Geometry check sheet. Reference: the model listing, model coordinates, mm. A direction names the side the tool comes from. Give positions to 0.01 mm unless a question says otherwise; leave off trailing zeros. Order: outer loops, then holes, each group sorted by start corner. A loop starts at its lowest first (then second) coordinate and runs counter-clockwise, first axis right, second up.
from build123d import *

# Parameters (mm, degrees)
SKETCH1_R           = 31.75
BOSS_EXTRUDE1_DEPTH = 38.1
SKETCH2_R           = 19.05
CUT_EXTRUDE1_DEPTH  = 12.7
SKETCH3_R           = 19.05
CUT_EXTRUDE2_DEPTH  = 39.1
SKETCH4_R           = 22.86
CUT_EXTRUDE3_DEPTH  = 7.62


with BuildPart() as part:
    # Sketch1 → Boss-Extrude1 (new body)
    with BuildSketch(Plane.XY):
        Circle(SKETCH1_R)
    extrude(amount=BOSS_EXTRUDE1_DEPTH)

    # Sketch2 → Cut-Extrude1 (cut)
    with BuildSketch(Plane(origin=(0, 0, 0), x_dir=(-1, 0, 0), z_dir=(0, 0, -1))):
        Circle(SKETCH2_R)
    extrude(amount=-CUT_EXTRUDE1_DEPTH, mode=Mode.SUBTRACT)

    # Sketch3 → Cut-Extrude2 (cut, through all)
    with BuildSketch(Plane.XY.offset(38.1)):
        with Locations(Location((0, 0, 0), (0, 0, 180))):  # turned: the seam where the file's is
            Circle(SKETCH3_R)
    extrude(amount=-CUT_EXTRUDE2_DEPTH, mode=Mode.SUBTRACT)

    # Sketch4 → Cut-Extrude3 (cut)
    with BuildSketch(Plane(origin=(0, 0, 0), x_dir=(-1, 0, 0), z_dir=(0, 0, -1))):
        Circle(SKETCH4_R)
    extrude(amount=-CUT_EXTRUDE3_DEPTH, mode=Mode.SUBTRACT)


solid = part.part
Item 1: Sectioned sample at A-A (y = 0). Enter the section's corners in (x, z).
Reported:
outline: (-31.75, 0) - (-22.86, 0) - (-22.86, 7.62) - (-19.05, 7.62) - (-19.05, 38.1) - (-31.75, 38.1) - close; (19.05, 7.62) - (22.86, 7.62) - (22.86, 0) - (31.75, 0) - (31.75, 38.1) - (19.05, 38.1) - close
Item 2: Draft check along X on faces 1 (the cylindrical face through (-6.883, -30.995, 18.783)), 2 (the flat face through (9, 17, 7.62)), 3 (the flat face through (-8, 22, 0)). Enter one of: released by +X, released by -X, zero draft, split by the parting line, or undercut.
Reported:
face 1: split by the parting line
face 2: undercut
face 3: zero draft
Item 3: Sectioned sample at C-C (z = 27.5). Enter the section's corners in (x, y).
Reported:
outline: circle Ø63.5 at (0, 0); hole circle Ø38.1 at (0, 0)
Item 4: Gauge pin test, flat ends, axial feed: pin 1 (8 mm diameter, centred on y = -20.5, z = 11, fed in from +X); pin 2 (4 mm diameter, centred on y = -15.5, z = 18, fed in from +X); pin 3 (3 mm diameter, centred on x = -15.5, z = 6.5, fed in from -Y). Record the tip position at first contact, or that the pin passes through.
Reported:
pin 1: stops at x = 27.13
pin 2: stops at x = 28.74
pin 3: stops at y = -28.5
Item 5: Set-up check for faces 4 (the cylindrical face through (-21.804, 6.867, 3.757)), 5 (the cylindrical face through (15.12, -11.59, 22.65)): record each of +Z, -Z, +X, -X, +Y, -Y from which the full face is reachable in a straight line by a thin tool's end or side.
Reported:
face 4: -Z
face 5: +Z, -Z
Item 6: Scan lines: L1, parallel to Y at x = 0, z = 4.5; L2, parallel to Y at x = 0, z = 18.5; L3, parallel to X at y = -15, z = 12. Record each from-to range of solid material in increasing order.
Reported:
L1: y = -31.75 to -22.86, 22.86 to 31.75
L2: y = -31.75 to -19.05, 19.05 to 31.75
L3: x = -27.98 to -11.74, 11.74 to 27.98
Item 7: Sectioned sample at D-D (x = -26). Enter the section's corners in (y, z), and give its area (3 significant figures).
Reported:
outline: (-18.22, 0) - (18.22, 0) - (18.22, 38.1) - (-18.22, 38.1) - close
area: 1,390 mm2
